CAD build for the part. Positions are in the model's coordinates, mm. Coordinates: 2 decimals unless noted, no trailing zeros. Write each loop counter-clockwise with the first axis right and the second up, starting at its lowest first coordinate (ties: lowest second). Pieces come first, ordered by that corner, then holes. Notation, with made-up numbers: (38.25, -38.75) - (58.25, -38.75) arc R19 ccw to (58.25, -27.75) - close; hole circle Ø11 at (61.25, 74). An arc over 180 degrees is marked (long way). Answer in a Markdown table with one row per item. Add a question column.
Q1. Pin check, flat tips, straight feed: pin 1 (7.5 mm diameter, centred on x = 1550, z = 9.5, fed in from +Y); pin 2 (4 mm diameter, centred on x = 1499, z = 8, fed in from +Y); pin 3 (7.5 mm diameter, centred on x = 1554, z = 13, fed in from -Y). Stop position of each tip, or through.
Q2. Band-saw the part on C-C (y = 1061). List the corners of the cut face in (x, z), and give its area (3 significant figures).
Q3. Band-saw the part on B-B (y = 1319). List the corners of the cut face in (x, z).
Q4. Drill centre lines: line 1 along X through (y, z) = (1771.5, 16.25); line 2 along X through (y, z) = (1285.5, 18); line 3 along Y through (x, z) = (1518, 3). Where is each one in solid material? Low to high. Write a range as from..to.
Q5. Band-saw the part on A-A (z = 5.5). State how many separate pieces and enclosed holes the cut face has, and give its area (3 significant figures).
```python
from build123d import *

# Parameters (mm, degrees)
SKETCH19_R          = 15.875
BOSS_EXTRUDE2_DEPTH = 19.05


with BuildPart() as part:
    # Sketch19 → Boss-Extrude2 (new body)
    with BuildSketch(Plane.XY):
        with BuildLine():
            add(Edge.make_bspline(
                [(1691.296561672, 1918.177904127), (1656.762851887, 2023.18607917), (1371.325091688, 2058.930160841), (1361.096561672, 1948.863494174)],
                knots=[0, 0, 0, 0, 7.638294788, 7.638294788, 7.638294788, 7.638294788], degree=3))
            Line((1361.096561672, 1948.863494174), (1361.096561672, 996.363494174))
            add(Edge.make_bspline(
                [(1691.296561672, 1027.049084222), (1656.707719979, 922.059056278), (1371.325091688, 886.296827508), (1361.096561672, 996.363494174)],
                knots=[0, 0, 0, 0, 7.629784399, 7.629784399, 7.629784399, 7.629784399], degree=3))
            ThreePointArc((1691.296561672, 1027.049084222), (1792.519416014, 1472.613494174), (1691.296561672, 1918.177904127))
        make_face()
        with BuildLine():
            Line((1556.504865632, 1122.44241392), (1547.43077252, 1122.44241392))
            Line((1547.43077252, 1122.44241392), (1547.43077252, 1112.28241392))
            ThreePointArc((1547.43077252, 1112.28241392), (1546.686823744, 1110.486362696), (1544.89077252, 1109.74241392))
            Line((1544.89077252, 1109.74241392), (1473.77077252, 1109.74241392))
            ThreePointArc((1473.77077252, 1109.74241392), (1471.974721296, 1110.486362696), (1471.23077252, 1112.28241392))
            Line((1471.23077252, 1112.28241392), (1471.23077252, 1122.44241392))
            Line((1471.23077252, 1122.44241392), (1459.984865632, 1122.44241392))
            ThreePointArc((1459.984865632, 1122.44241392), (1458.188814408, 1123.186362696), (1457.444865632, 1124.98241392))
            Line((1457.444865632, 1124.98241392), (1457.444865632, 1182.13241392))
            ThreePointArc((1457.444865632, 1182.13241392), (1458.188814408, 1183.928465145), (1459.984865632, 1184.67241392))
            Line((1459.984865632, 1184.67241392), (1471.23077252, 1184.67241392))
            Line((1471.23077252, 1184.67241392), (1471.23077252, 1188.48241392))
            ThreePointArc((1471.23077252, 1188.48241392), (1471.974721296, 1190.278465145), (1473.77077252, 1191.02241392))
            Line((1473.77077252, 1191.02241392), (1544.89077252, 1191.02241392))
            ThreePointArc((1544.89077252, 1191.02241392), (1546.686823744, 1190.278465145), (1547.43077252, 1188.48241392))
            Line((1547.43077252, 1188.48241392), (1547.43077252, 1184.67241392))
            Line((1547.43077252, 1184.67241392), (1556.504865632, 1184.67241392))
            ThreePointArc((1556.504865632, 1184.67241392), (1558.300916856, 1183.928465145), (1559.044865632, 1182.13241392))
            Line((1559.044865632, 1182.13241392), (1559.044865632, 1124.98241392))
            ThreePointArc((1559.044865632, 1124.98241392), (1558.300916856, 1123.186362696), (1556.504865632, 1122.44241392))
        make_face(mode=Mode.SUBTRACT)
        with BuildLine():
            Line((1444.893065071, 1244.244623225), (1435.893057671, 1279.244553225))
            ThreePointArc((1435.893057671, 1279.244553225), (1449.094985702, 1301.58631231), (1471.436744787, 1288.384384279))
            Line((1471.436744787, 1288.384384279), (1479.734522372, 1256.115340295))
            ThreePointArc((1479.734522372, 1256.115340295), (1479.841246759, 1255.791962976), (1479.990269115, 1255.485768066))
            Line((1479.990269115, 1255.485768066), (1495.595800102, 1228.231937145))
            ThreePointArc((1495.595800102, 1228.231937145), (1496.589194493, 1226.682766417), (1497.422422708, 1225.041884612))
            ThreePointArc((1497.422422708, 1225.041884612), (1488.994111708, 1201.213784587), (1464.764130707, 1208.40564094))
            Line((1464.764130707, 1208.40564094), (1446.764069078, 1239.655616711))
            ThreePointArc((1446.764069078, 1239.655616711), (1445.672935755, 1241.886666839), (1444.893065071, 1244.244623225))
        make_face(mode=Mode.SUBTRACT)
        with Locations(Location((1424.596561672, 1405.938494174, 0), (0, 0, 180))):
            Circle(SKETCH19_R, mode=Mode.SUBTRACT)
        with Locations(Location((1424.596561672, 1450.388494174, 0), (0, 0, 180))):
            Circle(SKETCH19_R, mode=Mode.SUBTRACT)
        with BuildLine():
            Line((1527.986726026, 1255.506514787), (1544.56575997, 1226.723451874))
            ThreePointArc((1544.56575997, 1226.723451874), (1537.823790218, 1201.663704337), (1512.764042681, 1208.405674089))
            Line((1512.764042681, 1208.405674089), (1494.764045881, 1239.655687936))
            ThreePointArc((1494.764045881, 1239.655687936), (1493.802589185, 1241.576837352), (1493.072252129, 1243.597189262))
            ThreePointArc((1493.072252129, 1243.597189262), (1492.894588833, 1244.238723731), (1492.740311476, 1244.886280075))
            Line((1492.740311476, 1244.886280075), (1483.894581433, 1279.238653731))
            ThreePointArc((1483.894581433, 1279.238653731), (1497.09201275, 1301.585586702), (1519.436740684, 1288.384422355))
            Line((1519.436740684, 1288.384422355), (1527.727745028, 1256.141718681))
            ThreePointArc((1527.727745028, 1256.141718681), (1527.835693423, 1255.815333734), (1527.986726026, 1255.506514787))
        make_face(mode=Mode.SUBTRACT)
        with Locations(Location((1424.596561672, 1494.838494174, 0), (0, 0, 180))):
            Circle(SKETCH19_R, mode=Mode.SUBTRACT)
        with Locations(Location((1424.596561672, 1539.288494174, 0), (0, 0, 180))):
            Circle(SKETCH19_R, mode=Mode.SUBTRACT)
        with BuildLine():
            Line((1547.43077252, 1681.24241392), (1547.43077252, 1671.08241392))
            ThreePointArc((1547.43077252, 1671.08241392), (1546.686823744, 1669.286362696), (1544.89077252, 1668.54241392))
            Line((1544.89077252, 1668.54241392), (1473.77077252, 1668.54241392))
            ThreePointArc((1473.77077252, 1668.54241392), (1471.974721296, 1669.286362696), (1471.23077252, 1671.08241392))
            Line((1471.23077252, 1671.08241392), (1471.23077252, 1681.24241392))
            Line((1471.23077252, 1681.24241392), (1459.984865632, 1681.24241392))
            ThreePointArc((1459.984865632, 1681.24241392), (1458.188814408, 1681.986362696), (1457.444865632, 1683.78241392))
            Line((1457.444865632, 1683.78241392), (1457.444865632, 1740.93241392))
            ThreePointArc((1457.444865632, 1740.93241392), (1458.188814408, 1742.728465145), (1459.984865632, 1743.47241392))
            Line((1459.984865632, 1743.47241392), (1471.23077252, 1743.47241392))
            Line((1471.23077252, 1743.47241392), (1471.23077252, 1747.28241392))
            ThreePointArc((1471.23077252, 1747.28241392), (1471.974721296, 1749.078465145), (1473.77077252, 1749.82241392))
            Line((1473.77077252, 1749.82241392), (1544.89077252, 1749.82241392))
            ThreePointArc((1544.89077252, 1749.82241392), (1546.686823744, 1749.078465145), (1547.43077252, 1747.28241392))
            Line((1547.43077252, 1747.28241392), (1547.43077252, 1743.47241392))
            Line((1547.43077252, 1743.47241392), (1556.504865632, 1743.47241392))
            ThreePointArc((1556.504865632, 1743.47241392), (1558.300916856, 1742.728465145), (1559.044865632, 1740.93241392))
            Line((1559.044865632, 1740.93241392), (1559.044865632, 1683.78241392))
            ThreePointArc((1559.044865632, 1683.78241392), (1558.300916856, 1681.986362696), (1556.504865632, 1681.24241392))
            Line((1556.504865632, 1681.24241392), (1547.43077252, 1681.24241392))
        make_face(mode=Mode.SUBTRACT)
        with BuildLine():
            Line((1444.893131568, 1803.044661302), (1435.893124168, 1838.044591302))
            ThreePointArc((1435.893124168, 1838.044591302), (1449.095052199, 1860.386350386), (1471.436811284, 1847.184422355))
            Line((1471.436811284, 1847.184422355), (1479.727821657, 1814.941695236))
            ThreePointArc((1479.727821657, 1814.941695236), (1479.835768961, 1814.615312965), (1479.98679977, 1814.30649635))
            Line((1479.98679977, 1814.30649635), (1496.565772911, 1785.52338757))
            ThreePointArc((1496.565772911, 1785.52338757), (1489.823779303, 1760.463721825), (1464.764105889, 1767.205686923))
            Line((1464.764105889, 1767.205686923), (1446.764116481, 1798.455687936))
            ThreePointArc((1446.764116481, 1798.455687936), (1445.672995031, 1800.686722627), (1444.893131568, 1803.044661302))
        make_face(mode=Mode.SUBTRACT)
        with BuildLine():
            Line((1492.893060968, 1803.044661302), (1483.893053568, 1838.044591302))
            ThreePointArc((1483.893053568, 1838.044591302), (1497.094981599, 1860.386350386), (1519.436740684, 1847.184422355))
            Line((1519.436740684, 1847.184422355), (1527.727745028, 1814.941718681))
            ThreePointArc((1527.727745028, 1814.941718681), (1527.835693423, 1814.615333734), (1527.986726026, 1814.306514787))
            Line((1527.986726026, 1814.306514787), (1544.56575257, 1785.523464721))
            ThreePointArc((1544.56575257, 1785.523464721), (1537.823782818, 1760.463717184), (1512.764035281, 1767.205686936))
            Line((1512.764035281, 1767.205686936), (1494.764045881, 1798.455687936))
            ThreePointArc((1494.764045881, 1798.455687936), (1493.672924431, 1800.686722627), (1492.893060968, 1803.044661302))
        make_face(mode=Mode.SUBTRACT)
    extrude(amount=BOSS_EXTRUDE2_DEPTH)


solid = part.part
```
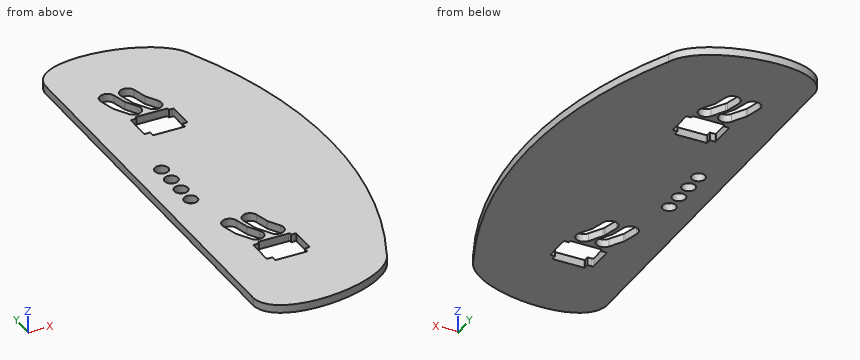
Checked values:
| question | item | result |
|---|---|---|
| 1 | pin 1 | stops at y = 2009.76 |
| 1 | pin 2 | stops at y = 2015.73 |
| 1 | pin 3 | stops at y = 936.28 |
| 2 | outline | (1361.1, 0) - (1706.81, 0) - (1706.81, 19.05) - (1361.1, 19.05) - close |
| 2 | area | 6,590 mm² |
| 3 | outline | (1361.1, 0) - (1781.01, 0) - (1781.01, 19.05) - (1361.1, 19.05) - close |
| 4 | line 1 | x = 1361.1..1462.29, 1498.36..1510.29, 1546.36..1748.26 |
| 4 | line 2 | x = 1361.1..1435.39, 1472.18..1483.39, 1520.18..1775.4 |
| 4 | line 3 | y = 931.16..1109.74, 1191.02..1202.63, 1292.17..1668.54, 1749.82..1761.43, 1850.97..2014.07 |
| 5 | separate pieces | 1 |
| 5 | enclosed holes | 10 |
| 5 | area | 372,000 mm² |
